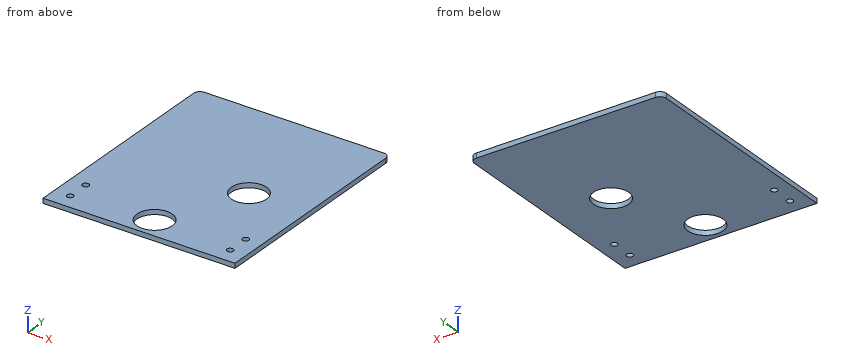
Autodesk Inventor part; units mm, degrees
ref_plane "YZ Plane" through (0, 0, 0) normal (1, 0, 0) x (0, 1, 0)
ref_plane "XZ Plane" through (0, 0, 0) normal (0, 1, 0) x (-1, 0, 0)
ref_plane "XY Plane" through (0, 0, 0) normal (0, 0, 1) x (1, 0, 0)
sketch "スケッチ1" plane through (0, 0, 0) normal (0, 0, 1) x (1, 0, 0)
  circle A0 centre (0, 0) radius 7.5
  circle A1 centre (0, 0) radius 30
  circle A2 centre (0, 0) radius 37.5
  circle A3 centre (23.5425, -29.1891) radius 30
  circle A4 centre (23.5425, -29.1891) radius 4
  circle A5 centre (23.5425, -29.1891) radius 16
  circle A6 centre (23.5425, -29.1891) radius 56
  circle A7 centre (0, -80) radius 40
  circle A8 centre (0, -80) radius 50
  circle A9 centre (0, -80) radius 4
  dimension "d57" = 75
  dimension "d64" = 112
  dimension "d41" = 15
  dimension "d58" = 8
  dimension "d63" = 32
  dimension "d65" = 100
  dimension "d66" = 8
sketch "スケッチ2" plane through (0, 0, 0) normal (0, 0, 1) x (1, 0, 0)
  line L0 (0, 0) -> (24.502, 0) construction
  line L1 (0, 0) -> (12.5, 0) construction
  line L2 (0, 0) -> (10.253, 10.253)
  line L3 (0, 0) -> (14.5, 0) construction
  line L4 (10.253, 10.253) -> (-10.253, -10.253)
  circle A0 centre (10.253, 10.253) radius 2
  circle A1 centre (-10.253, -10.253) radius 2
  circle A2 centre (0, 0) radius 7.5
  line L5 (0, 0) -> (28.1908, 10.2606)
  line L6 (0, 0) -> (30, 0) construction
  line L7 (0, 0) -> (-28.1908, 10.2606)
  line L8 (0, 0) -> (30, 0) construction
  circle A3 centre (-28.1908, 10.2606) radius 2.5
  line L9 (0, 0) -> (0, 30)
  circle A4 centre (0, 30) radius 2.5
  circle A5 centre (28.1908, 10.2606) radius 2.5
  dimension "d9" = 14.5
  dimension "d10" = 45
  dimension "d11" = 29
  dimension "d12" = 4
  dimension "d13" = 4
  dimension "d14" = 15
  dimension "d15" = 30
  dimension "d16" = 20
  dimension "d17" = 30
  dimension "d18" = 160
  dimension "d19" = 5
  dimension "d20" = 30
  dimension "d21" = 5
  dimension "d22" = 5
sketch "スケッチ3" plane through (0, 0, 0) normal (0, 0, 1) x (1, 0, 0)
  line L0 (60, -99.3436) -> (-60, -99.3436)
  line L1 (-60, -99.3436) -> (-60, 99.3436)
  line L2 (-60, 99.3436) -> (60, 99.3436)
  line L3 (60, 99.3436) -> (60, -99.3436)
  line L4 (60, -99.3436) -> (-60, 99.3436) construction
  line L5 (-60, -99.3436) -> (60, 99.3436) construction
  point P0 (0, 0)
  dimension "d25" = 120
extrude "押し出し1" add sketch "スケッチ3" against normal blind 3
sketch "スケッチ4" plane through (0, 0, 0) normal (0, 0, 1) x (1, 0, 0)
  line L0 (0, 45.0711) -> (68.3595, 45.0711)
  line L1 (68.3595, 45.0711) -> (-74.3824, 45.0711)
  line L2 (-74.3824, 45.0711) -> (108.1656, 45.0711)
  line L3 (108.1656, 45.0711) -> (108.1656, 129.4154)
  line L4 (108.1656, 129.4154) -> (-74.3824, 129.4154)
  line L5 (-74.3824, 129.4154) -> (-74.3824, 45.0711)
  point P0 (0, 0)
extrude "押し出し4" cut sketch "スケッチ4" against normal blind 10
fillet "フィレット1" radius 4 4 edges at (-60, 45.0711, -1.5) (60, 45.0711, -1.5) (-60, -99.3436, -1.5) (60, -99.3436, -1.5)
extrude "押し出し9" cut sketch "スケッチ1" against normal blind 10 contours A4 A2 | A2 A4 | A9 A6 | A6 A9
sketch "スケッチ8" plane through (0, 0, 0) normal (0, 0, 1) x (1, 0, 0)
  line L0 (-265.6992, -158.784) -> (100.3409, -158.784)
  line L1 (100.3409, -158.784) -> (100.3409, -94)
  line L2 (100.3409, -94) -> (-265.6992, -94)
  line L3 (-265.6992, -94) -> (-265.6992, -158.784)
  line L4 (-265.6992, -158.784) -> (100.3409, -94) construction
  line L5 (100.3409, -158.784) -> (-265.6992, -94) construction
  point P0 (0, 0)
  point P1 (0, -94)
  point P2 (-82.6791, -126.392)
extrude "押し出し10" cut sketch "スケッチ8" against normal blind 10
sketch "スケッチ9" plane through (0, 0, 0) normal (0, 0, 1) x (1, 0, 0)
  circle A0 centre (-50, -84) radius 2
  circle A1 centre (50, -84) radius 2
  circle A2 centre (-50, -70) radius 2
  circle A3 centre (50, -70) radius 2
  point P0 (0, 0)
  dimension "d73" = 4
  dimension "d74" = 4
  dimension "d75" = 4
  dimension "d76" = 4
extrude "押し出し12" cut sketch "スケッチ9" against normal blind 10
sketch "スケッチ10" plane through (0, 0, -3) normal (0, 0, -1) x (-1, 0, 0)
  circle A0 centre (-23.5425, -29.1891) radius 4
  circle A1 centre (-23.5425, -29.1891) radius 11
  circle A2 centre (0, -80) radius 4
  circle A3 centre (0, -80) radius 11
  point P0 (0, 0)
  dimension "d79" = 22
  dimension "d80" = 22
extrude "押し出し13" cut sketch "スケッチ10" against normal blind 10
properties part number "板3" material "アルミニウム 6061"
Geometry check sheet. Reference: the model listing, model coordinates, mm. Round coordinates to 2 decimals unless told otherwise and drop trailing zeros. Order: outer loops, then holes, each group sorted by start corner. A loop starts at its lowest first (then second) coordinate and runs counter-clockwise, first axis right, second up. Notation, with made-up numbers: (15, -0.5) -> (49, -0.5) arc R23 cw to (49, 37.5) -> close; hole circle Ø3 at (83, 53). An arc over 180 degrees is marked (long way). Return JSON: item names as keys, results as strings. Group by question number.
Q1. Material ranges on probe 1 along Y at (x, z) = (50, -1.25); probe 2 along Y at (x, z) = (26, -2.25); probe 3 along X at (y, z) = (-88, -2.45), recorded low to high. Write a range as from..to.
Q2. Section check B-B, the plane y = -80. Record the boundary of the cut face in (x, z).
Q3. Section check A-A, the plane x = -50. Record the boundary of the cut face in (y, z), plus the area to 3 significant figures.
Q4. Section check D-D, the plane z = -1. Record the boundary of the cut face in (x, y), plus the area to 3 significant figures.
Q5. Section check C-C, the plane x = 0. Record the boundary of the cut face in (y, z).
Numbers:
{
 "1": {"probe 1": "-94..-86, -82..-72, -68..45.07", "probe 2": "-94..-39.91, -18.47..45.07", "probe 3": "-60..-7.55, 7.55..60"},
 "2": {"outline": "(-60, -3) -> (-11, -3) -> (-11, 0) -> (-60, 0) -> close; (11, -3) -> (60, -3) -> (60, 0) -> (11, 0) -> close"},
 "3": {"outline": "(-94, -3) -> (-86, -3) -> (-86, 0) -> (-94, 0) -> close; (-82, -3) -> (-72, -3) -> (-72, 0) -> (-82, 0) -> close; (-68, -3) -> (45.07, -3) -> (45.07, 0) -> (-68, 0) -> close", "area": "393 mm^2"},
 "4": {"outline": "(-60, -94) -> (60, -94) -> (60, 41.07) arc R4 ccw to (56, 45.07) -> (-56, 45.07) arc R4 ccw to (-60, 41.07) -> close; hole circle Ø4 at (-50, -84); hole circle Ø4 at (-50, -70); hole circle Ø22 at (0, -80); hole circle Ø22 at (23.54, -29.19); hole circle Ø4 at (50, -84); hole circle Ø4 at (50, -70)", "area": "15,900 mm^2"},
 "5": {"outline": "(-94, -3) -> (-91, -3) -> (-91, 0) -> (-94, 0) -> close; (-69, -3) -> (45.07, -3) -> (45.07, 0) -> (-69, 0) -> close"}
}
